The listing builds one solid part. Answer for the finished solid, in the listing's coordinates (mm). Face numbers are marked on the shaded views. A direction names the side the tool comes from. Round coordinates to 2 decimals unless told otherwise and drop trailing zeros. Write each loop counter-clockwise with the first axis right and the second up, starting at its lowest first coordinate (ties: lowest second). Pieces come first, ordered by that corner, then holes.
(1) A cutting plane is placed at D-D, the plane z = 7.5. Give the vertices of the cut face in (x, y), and give its area (3 significant figures).
(2) A cutting plane is placed at B-B, the plane z = 2.5. Give the vertices of the cut face in (x, y), and give its area (3 significant figures).
(3) Each of these flat-tipped pins is pushed along its axis until it touches: pin 1 Ø1 at (x, z) = (-32.5, 10) entering from +Y; pin 2 Ø9 at (x, y) = (-24.65, -28.5) entering from -Z; pin 3 Ø1 at (y, z) = (18.5, 1.5) entering from +X; pin 4 Ø0.8 at (x, y) = (-29.5, 15) entering from +Z. Where does it stop, or does it pass through?
(4) The mould has two halves that part along Y. Classify the marked faces 1, 2 and 3: +Y half, -Y half, draft (parallel to the pull), parting line (faces both ways), or undercut.
(5) Find the intervals of material crossed by probe 1 along X at (y, z) = (-13.5, 2.25); probe 2 along X at (y, z) = (3, 5); probe 3 along X at (y, z) = (-28.5, 10), in increasing order.
(6) A cutting plane is placed at A-A, the plane y = -28.5. Give the vertices of the cut face in (x, z), and give its area (3 significant figures).
(7) A cutting plane is placed at C-C, the plane x = 11. Give the vertices of the cut face in (y, z).
(8) For the marked faces 4, 5 and 6, determine the directions among +Z, -Z, +X, -X, +Y, -Y from which every point of the face is accessible in a straight line to the end or side of a thin tool.
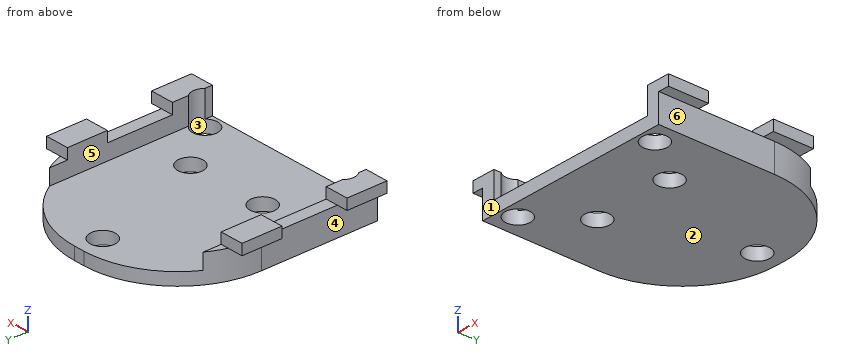
from build123d import *

# Parameters (mm, degrees)
F0_W         = 63.3
F0_H         = 67
F1_DEPTH     = 4
F3_W         = 4
F3_H         = 67
F4_DEPTH     = 5
F6_W         = 7.5
F6_H         = 12.75
F7_DEPTH     = 3.4
F2_R         = 4
F9_DEPTH     = 25
F8_R         = 4
F10_DEPTH    = 25
F11_T1_DEPTH = 84
F12_T1_DEPTH = 84


# Not quite as in the source:
# - a fillet or chamfer that OpenCascade refuses, or shapes differently, is made with other operations: its cross-section is extruded or revolved along the edge and cut away or added


with BuildPart() as f1:
    # F0 (on Top) → F1 (new body)
    with BuildSketch(Plane.XY):
        Rectangle(F0_W, F0_H)
    extrude(amount=F1_DEPTH)

    # F3 (on face) → F4 (join)
    with BuildSketch(Plane.XY.offset(4)):
        with Locations((-29.65, 0)):
            Rectangle(F3_W, F3_H)
        with Locations((29.65, 0)):
            Rectangle(F3_W, F3_H)
    extrude(amount=F4_DEPTH)

    # F6 (on face) → F7 (join)
    with BuildSketch(Plane.XY.offset(9)):
        with Locations((-31.4, 6.375)):
            Rectangle(F6_W, F6_H)
        with Locations((-31.4, -27.125)):
            Rectangle(F6_W, F6_H)
        with Locations((31.4, -27.125)):
            Rectangle(F6_W, F6_H)
        with Locations((31.4, 6.375)):
            Rectangle(F6_W, F6_H)
    extrude(amount=F7_DEPTH)

    # F2 (on Top) → F9 (cut)
    with BuildSketch(Plane.XY):
        with Locations((-24.65, -28.5)):
            Circle(F2_R)
        with Locations((24.65, -28.5)):
            Circle(F2_R)
    extrude(amount=F9_DEPTH, mode=Mode.SUBTRACT)

    # F8 (on Top) → F10 (cut)
    with BuildSketch(Plane.XY):
        with Locations((0, 26)):
            Circle(F8_R)
        with Locations((-13, -13.5)):
            Circle(F8_R)
        with Locations((13, -13.5)):
            Circle(F8_R)
    extrude(amount=F10_DEPTH, mode=Mode.SUBTRACT)

    # F11: fillet of radius 30 on 1 edges, made by hand

    # F11_s2 → F11_t1 (cut)
    with BuildSketch(Plane.XY.offset(-75)):
        with BuildLine():
            ThreePointArc((-1.65, 33.5), (-22.8632034356, 24.7132034356), (-31.65, 3.5))
            Line((-31.65, 3.5), (-31.65, 33.5))
            Line((-31.65, 33.5), (-1.65, 33.5))
        make_face()
    extrude(amount=F11_T1_DEPTH, mode=Mode.SUBTRACT)

    # F12: fillet of radius 30 on 1 edges, made by hand

    # F12_s2 → F12_t1 (cut)
    with BuildSketch(Plane.XY.offset(-75)):
        with BuildLine():
            ThreePointArc((31.65, 3.5), (22.8632034356, 24.7132034356), (1.65, 33.5))
            Line((1.65, 33.5), (31.65, 33.5))
            Line((31.65, 33.5), (31.65, 3.5))
        make_face()
    extrude(amount=F12_T1_DEPTH, mode=Mode.SUBTRACT)


solid = f1.part
Solutions:
1. outline: (-31.65, -33.5) - (-27.65, -33.5) - (-27.65, -31.15) arc R4 cw to (-27.65, -25.85) - (-27.65, 18.47) arc R30 ccw to (-31.65, 3.5) - close; (27.65, -33.5) - (31.65, -33.5) - (31.65, 3.5) arc R30 ccw to (27.65, 18.47) - (27.65, -25.85) arc R4 cw to (27.65, -31.15) - close
1. area: 370 mm2
2. outline: (-31.65, -33.5) - (31.65, -33.5) - (31.65, 3.5) arc R30 ccw to (1.65, 33.5) - (-1.65, 33.5) arc R30 ccw to (-31.65, 3.5) - close; hole circle Ø8 at (-24.65, -28.5); hole circle Ø8 at (-13, -13.5); hole circle Ø8 at (0, 26); hole circle Ø8 at (13, -13.5); hole circle Ø8 at (24.65, -28.5)
2. area: 3,600 mm2
3. pin 1: stops at y = 12.75
3. pin 2: stops at z = 0
3. pin 3: stops at x = 27.91
3. pin 4: stops at z = 9
4. face 1: -Y half
4. face 2: draft
4. face 3: undercut
5. probe 1: x = -31.65 to -17, -9 to 9, 17 to 31.65
5. probe 2: x = -31.65 to -27.65, 27.65 to 31.65
5. probe 3: x = -35.15 to -28.65, 28.65 to 35.15
6. outline: (-35.15, 9) - (-31.65, 9) - (-31.65, 0) - (-28.65, 0) - (-28.65, 12.4) - (-35.15, 12.4) - close; (-20.65, 0) - (20.65, 0) - (20.65, 4) - (-20.65, 4) - close; (28.65, 0) - (31.65, 0) - (31.65, 9) - (35.15, 9) - (35.15, 12.4) - (28.65, 12.4) - close
6. area: 263 mm2
7. outline: (-33.5, 0) - (-16.96, 0) - (-16.96, 4) - (-33.5, 4) - close; (-10.04, 0) - (32.01, 0) - (32.01, 4) - (-10.04, 4) - close
8. face 4: -Z, -X, +Y, -Y
8. face 5: +Z, +Y, -Y
8. face 6: -Z, +X, +Y, -Y
